Read the model definition and answer for the solid it produces. Units are mm, in the model's axes. Face numbers are marked on the shaded views. A direction names the side the tool comes from. Coordinates: 2 decimals unless noted, no trailing zeros. Write each loop counter-clockwise with the first axis right and the second up, starting at its lowest first coordinate (ties: lowest second). Pieces come first, ordered by that corner, then holes.
(1) Section B-B on y = 6.5 is taken. Write down the section's boundary in (x, z).
(2) Given pin 1 (2 mm diameter, centred on x = 1.5, z = 3.5, fed in from -Y); pin 2 (0.6 mm diameter, centred on x = 0, z = 0, fed in from +Y); pin 3 (2 mm diameter, centred on y = -2, z = 1.5, fed in from +X), each flat-ended and moving along its own axis, determine where each tip first touches the part or whether it passes through.
(3) Find the intervals of material crossed by probe 1 along X at (y, z) = (-2, 1.5); probe 2 along X at (y, z) = (4.5, 3); probe 3 along Z at (x, y) = (6.25, 0.25), in increasing order.
(4) The mould has two halves that part along X. Classify the marked faces 4, 5 and 6: +X half, -X half, draft (parallel to the pull), parting line (faces both ways), or undercut.
(5) Section A-A on z = -0.25 is taken. State how many separate pieces and enclosed holes the cut face has, then the cut area to 3 significant figures.
(6) Which of the six approach directions +Z, -Z, +X, -X, +Y, -Y give full straight-line access (tool end or side, diameter ignored) to the marked faces 1, 2 and 3?
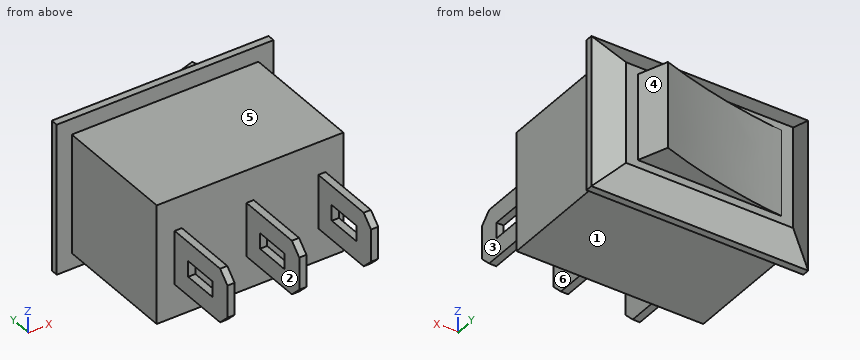
from build123d import *
from OCP.BRepFilletAPI import BRepFilletAPI_MakeChamfer

# Parameters (mm, degrees)
SKETCH1_W           = 13
SKETCH1_H           = 8.3
BOSS_EXTRUDE1_DEPTH = 8.65
SKETCH3_W           = 15.1
SKETCH3_H           = 10.5
BOSS_EXTRUDE2_DEPTH = 1.5
CHAMFER1_SIZE       = 1
CHAMFER1_SIZE2      = 1.732050808
SKETCH4_W           = 10
SKETCH4_H           = 6
BOSS_EXTRUDE3_DEPTH = 2
CUT_EXTRUDE2_DEPTH  = 6
SKETCH6_W           = 0.5
SKETCH6_H           = 3.75
BOSS_EXTRUDE4_DEPTH = 5.37
CHAMFER2_SIZE       = 0.75
CUT_EXTRUDE3_REACH  = 20.413
SKETCH7_W           = 1.1
SKETCH7_H           = 2.5


with BuildPart() as part:
    # Sketch1 → Boss-Extrude1 (new body)
    with BuildSketch(Plane(origin=(0, 0, 0), x_dir=(1, 0, 0), z_dir=(0, 1, 0))):
        Rectangle(SKETCH1_W, SKETCH1_H)
    extrude(amount=BOSS_EXTRUDE1_DEPTH)

    # Sketch3 → Boss-Extrude2 (add)
    with BuildSketch(Plane(origin=(0, 8.65, 0), x_dir=(1, 0, 0), z_dir=(0, 1, 0))):
        Rectangle(SKETCH3_W, SKETCH3_H)
    extrude(amount=BOSS_EXTRUDE2_DEPTH)

    # Chamfer1: one chamfer whose edges measure the first distance from different faces: ONE call of the kernel's chamfer builder (chamfer() names one face for all edges)
    chamfer1_edges_1 = [part.edges().sort_by_distance(p)[0] for p in [
        (-7.55, 10.15, 0),
    ]]
    chamfer1_side_1 = [part.faces().sort_by_distance(p)[0] for p in [
        (-7.55, 9.4, 0),
    ]]
    chamfer1_edges_2 = [part.edges().sort_by_distance(p)[0] for p in [
        (0, 10.15, 5.25),
    ]]
    chamfer1_side_2 = [part.faces().sort_by_distance(p)[0] for p in [
        (0, 9.4, 5.25),
    ]]
    chamfer1_edges_3 = [part.edges().sort_by_distance(p)[0] for p in [
        (7.55, 10.15, 0),
    ]]
    chamfer1_side_3 = [part.faces().sort_by_distance(p)[0] for p in [
        (7.55, 9.4, 0),
    ]]
    chamfer1_edges_4 = [part.edges().sort_by_distance(p)[0] for p in [
        (0, 10.15, -5.25),
    ]]
    chamfer1_side_4 = [part.faces().sort_by_distance(p)[0] for p in [
        (0, 9.4, -5.25),
    ]]
    chamfer1 = BRepFilletAPI_MakeChamfer(part.part.solid().wrapped)
    for e in chamfer1_edges_1:
        chamfer1.Add(CHAMFER1_SIZE, CHAMFER1_SIZE2, e.wrapped, chamfer1_side_1[0].wrapped)  # the first distance lies on this face
    for e in chamfer1_edges_2:
        chamfer1.Add(CHAMFER1_SIZE, CHAMFER1_SIZE2, e.wrapped, chamfer1_side_2[0].wrapped)  # the first distance lies on this face
    for e in chamfer1_edges_3:
        chamfer1.Add(CHAMFER1_SIZE, CHAMFER1_SIZE2, e.wrapped, chamfer1_side_3[0].wrapped)  # the first distance lies on this face
    for e in chamfer1_edges_4:
        chamfer1.Add(CHAMFER1_SIZE, CHAMFER1_SIZE2, e.wrapped, chamfer1_side_4[0].wrapped)  # the first distance lies on this face
    add(Compound.cast(chamfer1.Shape()), mode=Mode.REPLACE)

    # Sketch4 → Boss-Extrude3 (add)
    with BuildSketch(Plane(origin=(0, 10.15, 0), x_dir=(1, 0, 0), z_dir=(0, 1, 0))):
        Rectangle(SKETCH4_W, SKETCH4_H)
    extrude(amount=BOSS_EXTRUDE3_DEPTH)

    # Sketch5 → Cut-Extrude2 (cut)
    with BuildSketch(Plane(origin=(0, 0, -3), x_dir=(-1, 0, 0), z_dir=(0, 0, -1))):
        with BuildLine():
            Line((5, 12.15), (-4.272059531, 12.15))
            add(Edge.make_bspline(
                [(-4.272059531, 12.15), (0.251528144, 10.609590956), (5, 10.15)],
                knots=[0, 0, 0, 1, 1, 1], degree=2))
            Line((5, 10.15), (5, 12.15))
        make_face()
        Polygon((-5, 12.15), (-5, 10.15), (-4.272059531, 12.15), align=None)
    extrude(amount=-CUT_EXTRUDE2_DEPTH, mode=Mode.SUBTRACT)

    # Sketch6 → Boss-Extrude4 (add)
    with BuildSketch(Plane.XZ):
        Rectangle(SKETCH6_W, SKETCH6_H)
        with Locations((5, 0)):
            Rectangle(SKETCH6_W, SKETCH6_H)
        with Locations((-5, 0)):
            Rectangle(SKETCH6_W, SKETCH6_H)
    extrude(amount=BOSS_EXTRUDE4_DEPTH)

    # Chamfer2
    chamfer2_edges = [part.edges().sort_by_distance(p)[0] for p in [
        (0, -5.37, 1.875),
        (0, -5.37, -1.875),
        (5, -5.37, 1.875),
        (5, -5.37, -1.875),
        (-5, -5.37, 1.875),
        (-5, -5.37, -1.875),
    ]]
    chamfer(chamfer2_edges, length=CHAMFER2_SIZE)

    # Cut-Extrude3: up to this face of the body (flat: up to its plane)
    cut_extrude3_end = Plane(part.part.faces().sort_by_distance((5.25, -2.615028736, 0))[0])
    # Sketch7 → Cut-Extrude3 (cut, up to the picked face)
    with BuildSketch(Plane.ZY.offset(5.25), mode=Mode.PRIVATE) as cut_extrude3_sk1:
        with Locations((0, -2.62)):
            Rectangle(SKETCH7_W, SKETCH7_H)
    cut_extrude3_tool1 = split(extrude(cut_extrude3_sk1.sketch, amount=-CUT_EXTRUDE3_REACH, mode=Mode.PRIVATE), bisect_by=cut_extrude3_end, keep=Keep.BOTH, mode=Mode.PRIVATE)
    add(cut_extrude3_tool1.solids().sort_by(Axis((-5.25, -2.62, 0), (1, 0, 0)))[0], mode=Mode.SUBTRACT)


solid = part.part
Response:
1. outline: (-6.5, -4.15) - (6.5, -4.15) - (6.5, 4.15) - (-6.5, 4.15) - close
2. pin 1: stops at y = 0
2. pin 2: stops at y = 11.02
2. pin 3: stops at x = 5.25
3. probe 1: x = -5.25 to -4.75, -0.25 to 0.25, 4.75 to 5.25
3. probe 2: x = -6.5 to 6.5
3. probe 3: z = -4.15 to 4.15
4. face 4: +X half
4. face 5: draft
4. face 6: undercut
5. separate pieces: 4
5. enclosed holes: 0
5. area: 146 mm2
6. face 1: -Z, +X, -X, -Y
6. face 2: +Z, -Z, -Y
6. face 3: +Z, -Z, +X, -Y
